```python
from build123d import *

# Parameters (mm, degrees)
SKETCH1_W             = 50.8
SKETCH1_H             = 50.8
BOSS_EXTRUDE1_DEPTH   = 6.35
SKETCH2_R             = 1.5875
SKETCH2_R_2           = 3.175
BOSS_EXTRUDE2_DEPTH   = 25.4
F_4_40_TAPPED_HOLE1_D = 2.2606
FILLET1_R             = 0.635


with BuildPart() as part:
    # Sketch1 → Boss-Extrude1 (new body)
    with BuildSketch(Plane(origin=(0, 0, 0), x_dir=(0, 1, 0), z_dir=(0, 0, 1))):
        Rectangle(SKETCH1_W, SKETCH1_H)
    extrude(amount=BOSS_EXTRUDE1_DEPTH)

    # Sketch2 → Boss-Extrude2 (add)
    with BuildSketch(Plane.XY.offset(6.35)):
        with Locations(Location((0, -8.73125, 0), (0, 0, 180))):
            Circle(SKETCH2_R)
        with Locations(Location((0, 8.73125, 0), (0, 0, 180))):
            Circle(SKETCH2_R_2)
    extrude(amount=BOSS_EXTRUDE2_DEPTH)

    # #4-40 Tapped Hole1 (through all)
    with Locations(Plane.XY.offset(6.35)):
        with Locations((-20.32, -20.32), (-20.32, 20.32), (20.32, 20.32), (20.32, -20.32)):
            Hole(F_4_40_TAPPED_HOLE1_D / 2)

    # Fillet1
    fillet1_edges = [part.edges().sort_by_distance(p)[0] for p in [
        (0, -25.4, 6.35),
        (25.4, 0, 6.35),
        (0, 25.4, 6.35),
        (25.4, 0, 0),
        (0, -25.4, 0),
        (-25.4, 0, 0),
        (0, 25.4, 0),
        (25.4, 25.4, 3.175),
        (25.4, -25.4, 3.175),
        (-25.4, -25.4, 3.175),
        (-25.4, 25.4, 3.175),
        (-25.4, 0, 6.35),
    ]]
    fillet(fillet1_edges, radius=FILLET1_R)


solid = part.part
```
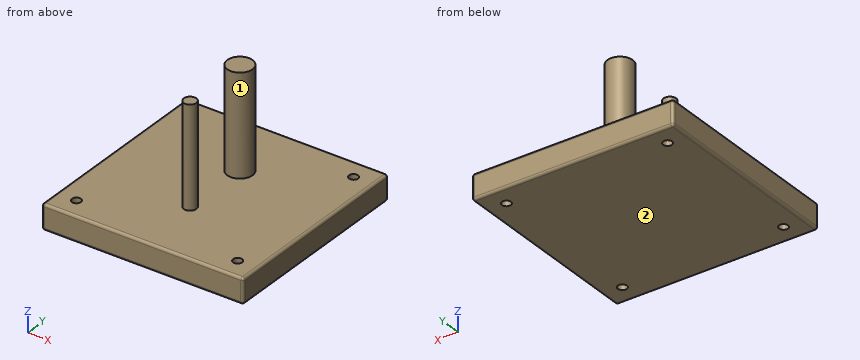
Input: part model. Units: mm. Frame: model coordinates. Face numbers are marked on the shaded views. A direction names the side the tool comes from. Coordinates: 2 decimals unless noted, no trailing zeros. Order: outer loops, then holes, each group sorted by start corner. A loop starts at its lowest first (then second) coordinate and runs counter-clockwise, first axis right, second up. Notation, with made-up numbers: (-21, -22.75) - (1, -22.75) arc R15 ccw to (1, -14.75) - close; hole circle Ø10 at (16.25, 18). An arc over 180 degrees is marked (long way). Put each result on its own line as item: value.
1. Line query: line 1 along Y through (x, z) = (-20.32, 4.5); line 2 along X through (y, z) = (20, 3); line 3 along Z through (x, y) = (-7.5, 20.5). Output: solid intervals per line, ascending.
Report:
line 1: y = -25.4 to -21.45, -19.19 to 19.19, 21.45 to 25.4
line 2: x = -25.4 to -21.4, -19.24 to 19.24, 21.4 to 25.4
line 3: z = 0 to 6.35
2. Cut plane B-B on x = 6. Return the cut outline in (y, z) (3 decimals).
Report:
outline: (-25.4, 0.635) arc R0.635 ccw to (-24.765, 0) - (24.765, 0) arc R0.635 ccw to (25.4, 0.635) - (25.4, 5.715) arc R0.635 ccw to (24.765, 6.35) - (-24.765, 6.35) arc R0.635 ccw to (-25.4, 5.715) - close
3. Contact query for flat-ended pins moving along their axis: pin 1 Ø5 at (x, y) = (14.5, -7.5) entering from -Z; pin 2 Ø1.4 at (x, y) = (20.32, 20.32) entering from -Z; pin 3 Ø3 at (x, y) = (-20.32, 20.32) entering from +Z. Output: stop coordinate, or through.
Report:
pin 1: stops at z = 0
pin 2: passes through
pin 3: stops at z = 6.35
4. Reachability of the marked faces 1 and 2 from +Z, -Z, +X, -X, +Y, -Y: full face, straight path, thin tool, end or side. Return the list, or none.
Report:
face 1: +Z
face 2: -Z, +X, -X, +Y, -Y
5. Cut plane A-A on y = -20.32. Return the cut outline in (x, z) (3 decimals), then the cut area to 3 significant figures.
Report:
outline: (-25.4, 0.635) arc R0.635 ccw to (-24.765, 0) - (-21.45, 0) - (-21.45, 6.35) - (-24.765, 6.35) arc R0.635 ccw to (-25.4, 5.715) - close; (-19.19, 0) - (19.19, 0) - (19.19, 6.35) - (-19.19, 6.35) - close; (21.45, 0) - (24.765, 0) arc R0.635 ccw to (25.4, 0.635) - (25.4, 5.715) arc R0.635 ccw to (24.765, 6.35) - (21.45, 6.35) - close
area: 294 mm2
